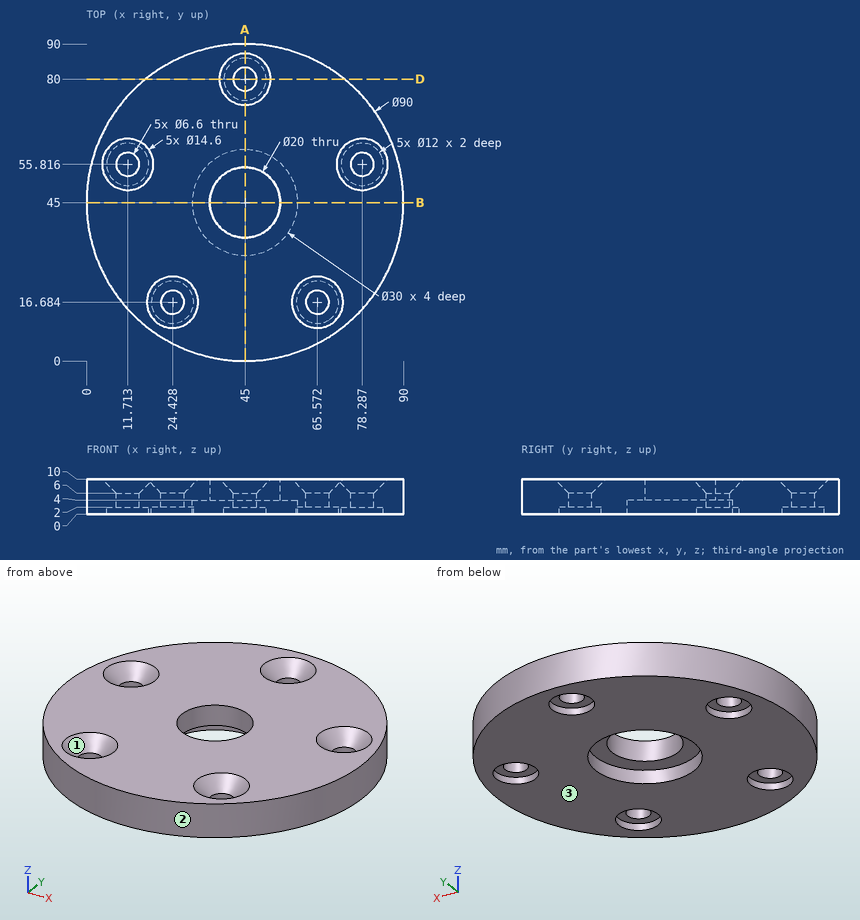
Here's the drawing with two shaded views (mm, measured from the low corner). I have some questions. Round coordinates to 2 decimals unless told otherwise and drop trailing zeros. Loops run counter-clockwise (first coordinate to the right, second up) from the corner with the lowest first, then second, coordinate; pieces in that order, holes last.
Item 1: Please list where these lines run through material, in increasing order: L1, parallel to Y at x = 45, z = 5.95; L2, parallel to Y at x = 45, z = 3.9; L3, parallel to X at y = 80.5, z = 6.5 (1 decimal).
Item 2: Suppose I cut it at D-D, the plane y = 80. Write out the boundary of the cut face in (x, z) (1 decimal).
Item 3: If we mould it in two halves opening along Y, with no side actions, what happens to the marked faces 1, 2 and 3? For each: +Y half, -Y half, draft (parallel to the pull), parting line (faces both ways), or undercut.
Item 4: Will these pins go through, and if not, where does the flat tip stop? pin 1 Ø3.5 at (x, y) = (42.5, 77.5) entering from -Z; pin 2 Ø9.5 at (x, y) = (78.29, 55.82) entering from +Z (1 decimal); pin 3 Ø3 at (x, z) = (71, 4.5) entering from -Y (1 decimal).
Item 5: Suppose I cut it at A-A, the plane x = 45. Write out the boundary of the cut face in (y, z), then the cut area to 3 significant figures.
Item 6: Suppose I cut it at B-B, the plane y = 45. Write out the boundary of the cut face in (x, z).
Reported:
1. L1: y = 0 to 35, 55 to 76.7, 83.3 to 90
1. L2: y = 0 to 30, 60 to 76.7, 83.3 to 90
1. L3: x = 17.3 to 41.2, 48.8 to 72.7
2. outline: (16.7, 0) - (39, 0) - (39, 2) - (41.7, 2) - (41.7, 6) - (37.7, 10) - (16.7, 10) - close; (48.3, 2) - (51, 2) - (51, 0) - (73.3, 0) - (73.3, 10) - (52.3, 10) - (48.3, 6) - close
3. face 1: undercut
3. face 2: parting line
3. face 3: draft
4. pin 1: stops at z = 2
4. pin 2: stops at z = 7.5
4. pin 3: stops at y = 7.3
5. outline: (0, 0) - (30, 0) - (30, 4) - (35, 4) - (35, 10) - (0, 10) - close; (55, 4) - (60, 4) - (60, 0) - (74, 0) - (74, 2) - (76.7, 2) - (76.7, 6) - (72.7, 10) - (55, 10) - close; (83.3, 2) - (86, 2) - (86, 0) - (90, 0) - (90, 10) - (87.3, 10) - (83.3, 6) - close
5. area: 567 mm2
6. outline: (0, 0) - (30, 0) - (30, 4) - (35, 4) - (35, 10) - (0, 10) - close; (55, 4) - (60, 4) - (60, 0) - (90, 0) - (90, 10) - (55, 10) - close
